from build123d import *

# Parameters (mm, degrees)
SKETCH1_R           = 50
BOSS_EXTRUDE1_DEPTH = 11
SKETCH2_R           = 30
CUT_EXTRUDE1_DEPTH  = 12
SKETCH3_W           = 150
SKETCH3_H           = 20
BOSS_EXTRUDE2_DEPTH = 20


with BuildPart() as part:
    # Sketch1 → Boss-Extrude1 (new, symmetric)
    with BuildSketch(Plane(origin=(0, 0, 0), x_dir=(0, 0, -1), z_dir=(1, 0, 0))):
        Circle(SKETCH1_R)
    extrude(amount=BOSS_EXTRUDE1_DEPTH, both=True)

    # Sketch2 → Cut-Extrude1 (cut)
    with BuildSketch(Plane.ZY.offset(11)):
        Circle(SKETCH2_R)
    extrude(amount=-CUT_EXTRUDE1_DEPTH, mode=Mode.SUBTRACT)

    # Sketch3 → Boss-Extrude2 (add)
    with BuildSketch(Plane(origin=(11, 0, 0), x_dir=(0, 0, -1), z_dir=(1, 0, 0))):
        Rectangle(SKETCH3_W, SKETCH3_H)
    extrude(amount=BOSS_EXTRUDE2_DEPTH)


solid = part.part
Work out the finished part from the listing and answer in its coordinate system (mm). A direction names the side the tool comes from. Give positions to 0.01 mm unless a question says otherwise; leave off trailing zeros. Order: outer loops, then holes, each group sorted by start corner. A loop starts at its lowest first (then second) coordinate and runs counter-clockwise, first axis right, second up. Notation, with made-up numbers: (62.25, 87) - (119.25, 87) arc R22 ccw to (119.25, 114) - close; hole circle Ø7 at (2.25, -39). An arc over 180 degrees is marked (long way). Answer as CSV lines item,"result". Start each with the question number.
Q1. The part is cut by section B-B (y = 0). Write down the section's boundary in (x, z), then the cut area to 3 significant figures.
Q2. The part is cut by section D-D (x = 23.5). Write down the section's boundary in (y, z), then the cut area to 3 significant figures.
Q3. Find the intervals of material crossed by L1, parallel to Y at x = -4.75, z = 0; L2, parallel to Y at x = 26.5, z = 7.5; L3, parallel to Z at x = -8.5, y = -16, in increasing order. Write a range as [from, to].
Q4. For faces 5 (the face through (11, 26, 1)), 6 (the face through (1, 0, 0)), 7 (the face through (11, -25, 1)), 8 (the face through (21, 0, -75)), determine the directions among +Z, -Z, +X, -X, +Y, -Y from which every point of the face is accessible in a straight line to the end or side of a thin tool.
Q5. Given pin 1 Ø6 at (x, z) = (26, -10) entering from -Y; pin 2 Ø22 at (y, z) = (-0.5, 65.5) entering from -X; pin 3 Ø10 at (x, z) = (24.5, -24.5) entering from +Y, each flat-ended and moving along its own axis, determine where each tip first touches the part or whether it passes through.
Q6. The mould has two halves that part along Z. Classify faces 1 (the face through (-5.08, 1.32, -29.97)), 2 (the face through (21, 0, 75)), 3 (the face through (21, 10, 1)), 4 (the face through (0.15, 15.02, -47.69)): +Z half, -Z half, draft (parallel to the pull), parting line (faces both ways), or undercut.
Q7. The part is cut by section A-A (z = 0). Write down the section's boundary in (x, y).
Q8. The part is cut by section C-C (x = -0.5). Write down the section's boundary in (y, z), then the cut area to 3 significant figures.
Check result:
1,outline,"(-11, -50) - (11, -50) - (11, -75) - (31, -75) - (31, 75) - (11, 75) - (11, 50) - (-11, 50) - (-11, 30) - (1, 30) - (1, -30) - (-11, -30) - close"
1,area,"4,480 mm²"
2,outline,"(-10, -75) - (10, -75) - (10, 75) - (-10, 75) - close"
2,area,"3,000 mm²"
3,L1,"y = [-50, -30], [30, 50]"
3,L2,"y = [-10, 10]"
3,L3,"z = [-47.37, -25.38], [25.38, 47.37]"
4,face 5,"+Z, -Z, +X, +Y"
4,face 6,"-X"
4,face 7,"+Z, -Z, +X, -Y"
4,face 8,"-Z, +X, -X, +Y, -Y"
5,pin 1,"stops at y = -10"
5,pin 2,"stops at x = 11"
5,pin 3,"stops at y = 10"
6,face 1,"undercut"
6,face 2,"+Z half"
6,face 3,"draft"
6,face 4,"parting line"
7,outline,"(-11, -50) - (11, -50) - (11, -10) - (31, -10) - (31, 10) - (11, 10) - (11, 50) - (-11, 50) - (-11, 30) - (1, 30) - (1, -30) - (-11, -30) - close"
8,outline,"circle Ø100 at (0, 0); hole circle Ø60 at (0, 0)"
8,area,"5,030 mm²"
